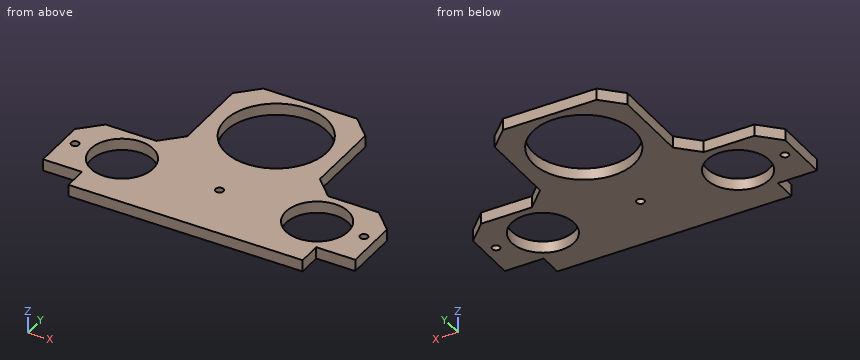
```python
from build123d import *

# Parameters (mm, degrees)
ESQUISSE1_R             = 13
BOSS_EXTRU_1_DEPTH      = 12
BOSS_EXTRU_2_START      = -12
ESQUISSE2_R             = 13
ESQUISSE2_R_2           = 5.5
BOSS_EXTRU_2_DEPTH      = 3
ESQUISSE4_R             = 8
ENL_V_MAT_EXTRU_2_DEPTH = 6
ESQUISSE5_R             = 3
ENL_V_MAT_EXTRU_3_DEPTH = 69.271516755
ENL_V_START             = -12
ESQUISSE6_W             = 10
ESQUISSE6_H             = 6
ENL_V_MAT_EXTRU_4_DEPTH = 12
CHANFREIN1_SIZE         = 5
ESQUISSE7_R             = 1
ENL_V_MAT_EXTRU_5_DEPTH = 12
ESQUISSE8_W             = 80
ESQUISSE8_H             = 3
ESQUISSE8_H_2           = 6
ENL_V_MAT_EXTRU_6_DEPTH = 70.057946682


with BuildPart() as part:
    # Esquisse1 → Boss.-Extru.1 (new body)
    with BuildSketch(Plane.XY):
        Polygon((-40, 0), (40, 0), (40, 25), (17, 25), (17, 55), (-17, 55), (-17, 25), (-40, 25), align=None)
        with Locations((0, 40)):
            Circle(ESQUISSE1_R, mode=Mode.SUBTRACT)
    extrude(amount=BOSS_EXTRU_1_DEPTH)

    # Esquisse2 → Boss.-Extru.2 (add)
    with BuildSketch(Plane.XY.offset(12).offset(BOSS_EXTRU_2_START)):
        with Locations((0, 40)):
            Circle(ESQUISSE2_R)
        with Locations((0, 40)):
            Circle(ESQUISSE2_R_2, mode=Mode.SUBTRACT)
    extrude(amount=BOSS_EXTRU_2_DEPTH)

    # Esquisse4 → Enlèv. mat.-Extru.2 (cut)
    with BuildSketch(Plane(origin=(0, 0, 0), x_dir=(-1, 0, 0), z_dir=(0, 0, -1))):
        with Locations((-25, 15)):
            Circle(ESQUISSE4_R)
        with Locations(Location((25, 15, 0), (0, 0, 180))):
            Circle(ESQUISSE4_R)
    extrude(amount=-ENL_V_MAT_EXTRU_2_DEPTH, mode=Mode.SUBTRACT)

    # Esquisse5 → Enlèv. mat.-Extru.3 (cut, through all)
    with BuildSketch(Plane(origin=(0, 0, 6), x_dir=(-1, 0, 0), z_dir=(0, 0, -1))):
        with Locations((-25, 15)):
            Circle(ESQUISSE5_R)
        with Locations(Location((25, 15, 0), (0, 0, 180))):
            Circle(ESQUISSE5_R)
    extrude(amount=-ENL_V_MAT_EXTRU_3_DEPTH, mode=Mode.SUBTRACT)

    # Esquisse6 → Enlèv. mat.-Extru.4 (cut)
    with BuildSketch(Plane.XY.offset(12).offset(ENL_V_START)):
        with Locations((35, 3)):
            Rectangle(ESQUISSE6_W, ESQUISSE6_H)
        with Locations((-35, 3)):
            Rectangle(ESQUISSE6_W, ESQUISSE6_H)
    extrude(amount=ENL_V_MAT_EXTRU_4_DEPTH, mode=Mode.SUBTRACT)

    # Chanfrein1
    chanfrein1_edges = [part.edges().sort_by_distance(p)[0] for p in [
        (-17, 55, 6),
        (17, 55, 6),
        (17, 25, 6),
        (40, 25, 6),
        (-40, 25, 6),
        (-17, 25, 6),
    ]]
    chamfer(chanfrein1_edges, length=CHANFREIN1_SIZE)

    # Esquisse7 → Enlèv. mat.-Extru.5 (cut)
    with BuildSketch(Plane(origin=(0, 0, 0), x_dir=(-1, 0, 0), z_dir=(0, 0, -1))):
        with Locations((-10, 45)):
            Circle(ESQUISSE7_R)
        with Locations(Location((10, 45, 0), (0, 0, 180))):
            Circle(ESQUISSE7_R)
        with Locations((-37, 15)):
            Circle(ESQUISSE7_R)
        with Locations(Location((37, 15, 0), (0, 0, 180))):
            Circle(ESQUISSE7_R)
        with Locations((0, 15)):
            Circle(ESQUISSE7_R)
    extrude(amount=-ENL_V_MAT_EXTRU_5_DEPTH, mode=Mode.SUBTRACT)

    # Esquisse8 → Enlèv. mat.-Extru.6 (cut, through all)
    with BuildSketch(Plane(origin=(0, 55, 0), x_dir=(1, 0, 0), z_dir=(0, 1, 0))):
        with Locations((0, -1.5)):
            Rectangle(ESQUISSE8_W, ESQUISSE8_H)
        with Locations((0, -9)):
            Rectangle(ESQUISSE8_W, ESQUISSE8_H_2)
    extrude(amount=-ENL_V_MAT_EXTRU_6_DEPTH, mode=Mode.SUBTRACT)


solid = part.part
```
The listing builds one solid part. Answer for the finished solid, in the listing's coordinates (mm). Round coordinates to 2 decimals unless told otherwise and drop trailing zeros. Loops run counter-clockwise (first coordinate to the right, second up) from the corner with the lowest first, then second, coordinate; pieces in that order, holes last.
Q1. Section A-A, the plane x = 25 is taken. Determine the outline of the cut face in (y, z).
Q2. Find the intervals of material crossed by line 1 (Y direction, x = 0, z = 4.95); line 2 (X direction, y = 10.5, z = 4.1); line 3 (X direction, y = 9.5, z = 5.2), in increasing order.
Q3. Section B-B, the plane z = 4.75 is taken. Determine the outline of the cut face in (x, y), then the cut area to 3 significant figures.
Q4. Section C-C, the plane y = 40 is taken. Determine the outline of the cut face in (x, z), then the cut area to 3 significant figures.
Q5. Given pin 1 Ø0.9 at (x, z) = (-31, 4) entering from +Y; pin 2 Ø15.5 at (x, y) = (0, 40) entering from +Z; pin 3 Ø1.5 at (y, z) = (35, 4.5) entering from -X; pin 4 Ø1.5 at (x, z) = (-37, 5) entering from -Y, each flat-ended and moving along its own axis, determine where each tip first touches the part or whether it passes through.
Q6. Section D-D, the plane x = 0 is taken. Determine the outline of the cut face in (y, z), then the cut area to 3 significant figures.
Completed:
1. outline: (0, 3) - (7, 3) - (7, 6) - (0, 6) - close; (23, 3) - (25, 3) - (25, 6) - (23, 6) - close
2. line 1: y = 0 to 14, 16 to 27, 53 to 55
2. line 2: x = -40 to -31.61, -18.39 to 18.39, 31.61 to 40
2. line 3: x = -40 to -30.81, -19.19 to 19.19, 30.81 to 40
3. outline: (-40, 6) - (-30, 6) - (-30, 0) - (30, 0) - (30, 6) - (40, 6) - (40, 20) - (35, 25) - (22, 25) - (17, 30) - (17, 50) - (12, 55) - (-12, 55) - (-17, 50) - (-17, 30) - (-22, 25) - (-35, 25) - (-40, 20) - close; hole circle Ø2 at (-37, 15); hole circle Ø16 at (-25, 15); hole circle Ø26 at (0, 40); hole circle Ø2 at (0, 15); hole circle Ø16 at (25, 15); hole circle Ø2 at (37, 15)
3. area: 1,930 mm2
4. outline: (-17, 3) - (-13, 3) - (-13, 6) - (-17, 6) - close; (13, 3) - (17, 3) - (17, 6) - (13, 6) - close
4. area: 24.0 mm2
5. pin 1: stops at y = 25
5. pin 2: passes through
5. pin 3: stops at x = -17
5. pin 4: stops at y = 6
6. outline: (0, 3) - (14, 3) - (14, 6) - (0, 6) - close; (16, 3) - (27, 3) - (27, 6) - (16, 6) - close; (53, 3) - (55, 3) - (55, 6) - (53, 6) - close
6. area: 81.0 mm2
